Source: CAD feature listing. Evaluate the final solid. Frame: model axes, mm. A direction names the side the tool comes from. Give positions to 0.01 mm unless a question says otherwise; leave off trailing zeros. Loops run counter-clockwise (first coordinate to the right, second up) from the corner with the lowest first, then second, coordinate; pieces in that order, holes last. Notation, with made-up numbers: (9, -2.5) - (17, -2.5) arc R19 ccw to (17, 4.5) - close; hole circle Ø11 at (-10, -36). An arc over 180 degrees is marked (long way). Write each question's results on one line, items separated by ' | '. Start each with the question number.
(1) Cut plane A-A on y = 2.7. Return the cut outline in (x, z), then the cut area to 3 significant figures.
(2) Contact query for a flat-ended pin moving along its axis: pin 1 (1 mm diameter, centred on y = 3, z = -8.5, fed in from -X). Output: stop coordinate, or through.
(3) Cut plane B-B on x = 10. Return the cut outline in (y, z), then the cut area to 3 significant figures.
(4) Cut plane C-C on z = -16.5. Return the cut outline in (x, y).
(5) Reachability of faces 4 (the flat face through (-2, 3, -21)), 5 (the flat face through (0, 2, 23)) from +Z, -Z, +X, -X, +Y, -Y: full face, straight path, thin tool, end or side. Return the list, or none.
(6) Pull-direction query (Z, two-part tool) for faces 1 (the cylindrical face through (20.4, 2.03, 22.43)), 2 (the flat face through (18, 3, -11)), 3 (the flat face through (0, 0, 0)); classes: pulls with the +Z half, pulls with the -Z half, needs draft (parallel to the pull), parting line crosses it, or undercut.
(7) Material intervals for line 1 along Z through (x, y) = (1.5, 3); line 2 along Y through (x, z) = (-14.5, -6); line 3 along X through (y, z) = (3.1, -4.5), sorted ascending. Write a range as [from, to].
Autodesk Inventor part; units mm, degrees
ref_plane "YZ Plane" through (0, 0, 0) normal (1, 0, 0) x (0, 1, 0)
ref_plane "XZ Plane" through (0, 0, 0) normal (0, 1, 0) x (-1, 0, 0)
ref_plane "XY Plane" through (0, 0, 0) normal (0, 0, 1) x (1, 0, 0)
sketch "Sketch1" plane through (0, 0, 0) normal (0, 1, 0) x (-1, 0, 0)
  line L0 (-21, 23) -> (21, 23)
  line L1 (21, 23) -> (21, -23)
  line L2 (21, -23) -> (-21, -23)
  line L3 (-21, -23) -> (-21, 23)
  line L4 (-21, 23) -> (21, -23) construction
  line L5 (21, 23) -> (-21, -23) construction
  point P0 (0, 0)
  dimension "d0" = 42
  dimension "d1" = 46
extrude "wall3" add sketch "Sketch1" along normal blind 4
fillet "Fillet6" radius 2 1 edges at (-21, 2, -23)
fillet "Fillet7" radius 2 1 edges at (21, 2, -23)
fillet "Fillet8" radius 2 1 edges at (-21, 2, 23)
fillet "Fillet9" radius 2 1 edges at (21, 2, 23)
sketch "Sketch10" plane through (0, 4, 0) normal (0, 1, 0) x (1, 0, 0)
  line L0 (-20.8799, 11) -> (21, 11) construction
  line L1 (21, -21) -> (21, 21)
  line L2 (14.0018, 23) -> (14.0018, -23) construction
  line L3 (-19, -23) -> (19, -23)
  line L4 (19, 23) -> (-19, 23)
  line L5 (-21, 21) -> (18, 21)
  line L6 (18, 21) -> (18, 1)
  line L7 (18, 1) -> (-21, 1)
  line L8 (-21, 1) -> (-21, 21)
  line L9 (-21, 21) -> (18, 1) construction
  line L10 (18, 21) -> (-21, 1) construction
  line L11 (-21, 21) -> (-21, -21)
  point P0 (0, 0)
  point P1 (-1.5, 11)
  dimension "d98" = 34
  dimension "d99" = 20
  dimension "d100" = 3
extrude "Extrusion8" cut sketch "Sketch10" against normal blind 2
equation "\"d0\" = wallw"
equation "\"d72\" = wall3_thick"
equation "\"d89\" = cornerrad"
equation "\"d90\" = cornerrad"
equation "\"d91\" = cornerrad"
equation "\"d92\" = cornerrad"
equation "\"d98\" = distancefrombottom"
equation "\"d99\" = wall3sloth"
equation "\"d100\" = -0.5 * wall3slotw + 0.5 * wallw"
equation "\"d101\" = wall3slotd"
equation "\"printer3dtolerance\" = 0.12"
equation "\"wallw\" = 42"
equation "\"wallh\" = 44"
equation "\"cornerrad\" = 2"
equation "\"baseextra\" = 2"
equation "\"wall1_thick\" = 8"
equation "\"wall2_thick\" = 6.4"
equation "\"wall3_thick\" = 4"
equation "\"wall1slot\" = 8.12"
equation "\"wall2slot\" = 6.52"
equation "\"wall3slot\" = 4.12"
equation "\"gap2\" = 28"
equation "\"baseh\" = 79.12"
equation "\"basew\" = 44"
equation "\"base_thick\" = 6"
equation "\"base_slots_depth\" = 4"
equation "\"servomounth\" = 4"
equation "\"servosmallcircledia\" = 5.92"
equation "\"servomountsquare\" = 6"
equation "\"servobigcircledia\" = 11.62"
equation "\"servo9gw\" = 22.8"
equation "\"distancefromleft\" = 26"
equation "\"servopolygonl\" = 5.92"
equation "\"servopolygonr\" = 6.12"
equation "\"distancefrombottom\" = 34"
equation "\"d49\" = distancefrombottom"
equation "\"adapterh\" = 16"
equation "\"adapterw\" = 32"
equation "\"wall3sloth\" = 20"
equation "\"wall3slotw\" = 36"
equation "\"wall3slotd\" = 2"
properties part number "wall-end" material "Wood (Oak)"
Ans:
1) outline: (-21, -21) arc R2 ccw to (-19, -23) - (19, -23) arc R2 ccw to (21, -21) - (21, 21) arc R2 ccw to (19, 23) - (-19, 23) arc R2 ccw to (-21, 21) - (-21, -1) - (18, -1) - (18, -21) - close | area: 1,150 mm^2
2) pin 1: x = 18
3) outline: (0, -23) - (4, -23) - (4, -21) - (2, -21) - (2, -1) - (4, -1) - (4, 23) - (0, 23) - close | area: 144 mm^2
4) outline: (-21, 0) - (21, 0) - (21, 4) - (18, 4) - (18, 2) - (-21, 2) - close
5) face 4: -X, +Y | face 5: +Z, +X, -X, +Y, -Y
6) face 1: pulls with the +Z half | face 2: undercut | face 3: needs draft
7) line 1: [-23, -21], [-1, 23] | line 2: [0, 2] | line 3: [18, 21]
